CAD build for the part. Positions are in the model's coordinates, mm. A direction names the side the tool comes from. Round coordinates to 2 decimals unless told otherwise and drop trailing zeros. Order: outer loops, then holes, each group sorted by start corner. A loop starts at its lowest first (then second) coordinate and runs counter-clockwise, first axis right, second up. Notation, with made-up numbers: (-21, 86) - (-4, 86) arc R22 ccw to (-4, 96) - close; hole circle Ø2 at (-23, 30). An arc over 180 degrees is marked (long way). Write item = value, one per line.
from build123d import *

# Parameters (mm, degrees)
CUT_EXTRUDE1_REACH = 247.25
SKETCH3_R          = 0.80645


with BuildPart() as part:
    # Sketch1 → Revolve1 (revolve)
    with BuildSketch(Plane.XY, mode=Mode.PRIVATE) as revolve1_sk:
        Polygon((0, 12.7), (196.85, 12.7), (196.85, 26.162), (241.3, 26.162), (241.3, 0), (259.36, 0), (259.36, 10.7696), (273.6661, 5.5626), (273.6661, 31), (0, 31), align=None)
    revolve(revolve1_sk.sketch.rotate(Axis((0, 0, 0), (1, 0, 0)), 90), axis=Axis((0, 0, 0), (1, 0, 0)))

    # Sketch3 → Cut-Extrude1 (cut, up to next)
    with BuildSketch(Plane.ZY.offset(-241.3), mode=Mode.PRIVATE) as cut_extrude1_sk1:
        with Locations((0, 6.477)):
            Circle(SKETCH3_R)
    cut_extrude1_tool1 = extrude(cut_extrude1_sk1.sketch, amount=-CUT_EXTRUDE1_REACH, mode=Mode.PRIVATE) & part.part
    # Sketch3 → Cut-Extrude1 (cut, up to next)
    with BuildSketch(Plane.ZY.offset(-241.3), mode=Mode.PRIVATE) as cut_extrude1_sk2:
        with Locations((4.579930622, 4.579930622)):
            Circle(SKETCH3_R)
    cut_extrude1_tool2 = extrude(cut_extrude1_sk2.sketch, amount=-CUT_EXTRUDE1_REACH, mode=Mode.PRIVATE) & part.part
    # Sketch3 → Cut-Extrude1 (cut, up to next)
    with BuildSketch(Plane.ZY.offset(-241.3), mode=Mode.PRIVATE) as cut_extrude1_sk3:
        with Locations((6.477, 0)):
            Circle(SKETCH3_R)
    cut_extrude1_tool3 = extrude(cut_extrude1_sk3.sketch, amount=-CUT_EXTRUDE1_REACH, mode=Mode.PRIVATE) & part.part
    # Sketch3 → Cut-Extrude1 (cut, up to next)
    with BuildSketch(Plane.ZY.offset(-241.3), mode=Mode.PRIVATE) as cut_extrude1_sk4:
        with Locations((4.579930622, -4.579930622)):
            Circle(SKETCH3_R)
    cut_extrude1_tool4 = extrude(cut_extrude1_sk4.sketch, amount=-CUT_EXTRUDE1_REACH, mode=Mode.PRIVATE) & part.part
    # Sketch3 → Cut-Extrude1 (cut, up to next)
    with BuildSketch(Plane.ZY.offset(-241.3), mode=Mode.PRIVATE) as cut_extrude1_sk5:
        with Locations((0, -6.477)):
            Circle(SKETCH3_R)
    cut_extrude1_tool5 = extrude(cut_extrude1_sk5.sketch, amount=-CUT_EXTRUDE1_REACH, mode=Mode.PRIVATE) & part.part
    # Sketch3 → Cut-Extrude1 (cut, up to next)
    with BuildSketch(Plane.ZY.offset(-241.3), mode=Mode.PRIVATE) as cut_extrude1_sk6:
        with Locations((-4.579930622, -4.579930622)):
            Circle(SKETCH3_R)
    cut_extrude1_tool6 = extrude(cut_extrude1_sk6.sketch, amount=-CUT_EXTRUDE1_REACH, mode=Mode.PRIVATE) & part.part
    # Sketch3 → Cut-Extrude1 (cut, up to next)
    with BuildSketch(Plane.ZY.offset(-241.3), mode=Mode.PRIVATE) as cut_extrude1_sk7:
        with Locations((-6.477, 0)):
            Circle(SKETCH3_R)
    cut_extrude1_tool7 = extrude(cut_extrude1_sk7.sketch, amount=-CUT_EXTRUDE1_REACH, mode=Mode.PRIVATE) & part.part
    # Sketch3 → Cut-Extrude1 (cut, up to next)
    with BuildSketch(Plane.ZY.offset(-241.3), mode=Mode.PRIVATE) as cut_extrude1_sk8:
        with Locations((-4.579930622, 4.579930622)):
            Circle(SKETCH3_R)
    cut_extrude1_tool8 = extrude(cut_extrude1_sk8.sketch, amount=-CUT_EXTRUDE1_REACH, mode=Mode.PRIVATE) & part.part
    add(cut_extrude1_tool1.solids().sort_by_distance((241.3, 6.477, 0))[0], mode=Mode.SUBTRACT)
    add(cut_extrude1_tool2.solids().sort_by_distance((241.3, 4.579931, 4.579931))[0], mode=Mode.SUBTRACT)
    add(cut_extrude1_tool3.solids().sort_by_distance((241.3, 0, 6.477))[0], mode=Mode.SUBTRACT)
    add(cut_extrude1_tool4.solids().sort_by_distance((241.3, -4.579931, 4.579931))[0], mode=Mode.SUBTRACT)
    add(cut_extrude1_tool5.solids().sort_by_distance((241.3, -6.477, 0))[0], mode=Mode.SUBTRACT)
    add(cut_extrude1_tool6.solids().sort_by_distance((241.3, -4.579931, -4.579931))[0], mode=Mode.SUBTRACT)
    add(cut_extrude1_tool7.solids().sort_by_distance((241.3, 0, -6.477))[0], mode=Mode.SUBTRACT)
    add(cut_extrude1_tool8.solids().sort_by_distance((241.3, 4.579931, -4.579931))[0], mode=Mode.SUBTRACT)


solid = part.part
(1) Band-saw the part on A-A on y = 21. List the corners of the cut face in (x, z).
Solved:
outline = (0, -22.8) - (273.67, -22.8) - (273.67, 22.8) - (0, 22.8) - close; hole (196.85, -15.6) - (241.3, -15.6) - (241.3, 15.6) - (196.85, 15.6) - close
(2) Drop flat-ended pins along their axis: pin 1 (2.5 mm diameter, centred on y = -6.477, z = 0, fed in from -X); pin 2 (12 mm diameter, centred on x = 217.5, z = 11, fed in from +Y); pin 3 (1 mm diameter, centred on x = 240, y = -16, fed in from +Z). Give the stop position or say it passes through.
Solved:
pin_1 = 241.3
pin_2 = 30.59
pin_3 = 26.85
(3) Band-saw the part on D-D on x = 74.5. List the corners of the cut face in (y, z), plus the area to 3 significant figures.
Solved:
outline = circle Ø62 at (0, 0); hole circle Ø25.4 at (0, 0)
area = 2,510 mm²
(4) Probe line 1 along X through (y, z) = (-15, -11); line 2 along Y through (x, z) = (68, 0); line 3 along X through (y, z) = (10.5, 7). List the from-to ranges inside material, lowest first.
Solved:
line_1 = 0 to 196.85, 241.3 to 273.67
line_2 = -31 to -12.7, 12.7 to 31
line_3 = 241.3 to 273.67
(5) Tool access for faces 1 (the conical face through (269.79, 6.81, -1.51)), 2 (the cylindrical face through (99.8, 7.7, -10.1)): list every direction of +Z, -Z, +X, -X, +Y, -Y with a clear straight run to the whole face (end or side of a thin tool).
Solved:
face_1 = none
face_2 = -X
(6) Pull direction X, two halves, no side cores. Call faces 3 (the flat face through (241.3, 0, 0)), 4 (the flat face through (0, 13, 0)), 5 (the flat face through (273.666, 6, 0)), 6 (the cylindrical face through (134.917, -30.736, -4.036)): released by +X, released by -X, zero draft, split by the parting line, or undercut.
Solved:
face_3 = undercut
face_4 = released by -X
face_5 = released by +X
face_6 = zero draft
(7) Band-saw the part on B-B on z = -15. List the corners of the cut face in (x, y).
Solved:
outline = (0, -27.13) - (273.67, -27.13) - (273.67, 27.13) - (0, 27.13) - close; hole (196.85, -21.43) - (241.3, -21.43) - (241.3, 21.43) - (196.85, 21.43) - close
(8) Band-saw the part on C-C on x = 208. List the corners of the cut face in (y, z).
Solved:
outline = circle Ø62 at (0, 0); hole circle Ø52.32 at (0, 0)
